Part model, mm, in its own coordinate system. A direction names the side the tool comes from. Round coordinates to 2 decimals unless told otherwise and drop trailing zeros. Order: outer loops, then holes, each group sorted by start corner. A loop starts at its lowest first (then second) coordinate and runs counter-clockwise, first axis right, second up. Notation, with made-up numbers: M 38.25,-31.5 L 88.25,-31.5 A6 cw 88.25,-27.5 Z; hole C 39,-24.75 d10. An arc over 180 degrees is marked long. One line per question, with ' | ' between items.
from build123d import *

# Parameters (mm, degrees)
F0_W     = 150
F0_H     = 125
F0_R     = 20
F1_DEPTH = 5
F2_R     = 10
F4_D     = 8.5
F4_DEPTH = 24.5
F4_TIP   = 2.5536576309
F6_DEPTH = 10.001


with BuildPart() as f1:
    # F0 (on Front) → F1 (new body, symmetric)
    with BuildSketch(Plane.XZ):
        Rectangle(F0_W, F0_H)
        Circle(F0_R, mode=Mode.SUBTRACT)
    extrude(amount=F1_DEPTH, both=True)

    # F2
    f2_edges = [f1.edges().sort_by_distance(p)[0] for p in [
        (-75, 0, 62.5),
        (75, 0, 62.5),
        (75, 0, -62.5),
        (-75, 0, -62.5),
    ]]
    fillet(f2_edges, radius=F2_R)

    # F4
    with Locations(Plane.XZ.offset(5)):
        with Locations((-49.5, 0), (49.5, 0)):
            Hole(F4_D / 2, depth=F4_DEPTH)
            with Locations((0, 0, -(F4_DEPTH + F4_TIP / 2))):  # 118° drill point
                Cone(0, F4_D / 2, F4_TIP, mode=Mode.SUBTRACT)

    # F5 (on face) → F6 (cut, through all)
    with BuildSketch(Plane.XZ.offset(5)):
        with BuildLine():
            ThreePointArc((-37.5, 53), (-43, 47.5), (-37.5, 42))
            Line((-37.5, 42), (37.5, 42))
            ThreePointArc((37.5, 42), (43, 47.5), (37.5, 53))
            Line((37.5, 53), (-37.5, 53))
        make_face()
        with BuildLine():
            ThreePointArc((37.5, -53), (43, -47.5), (37.5, -42))
            Line((37.5, -42), (-37.5, -42))
            ThreePointArc((-37.5, -42), (-43, -47.5), (-37.5, -53))
            Line((-37.5, -53), (37.5, -53))
        make_face()
    extrude(amount=-F6_DEPTH, mode=Mode.SUBTRACT)


solid = f1.part
1) Saw through at A-A (z = 47.5). List the corners of the cut face in (x, y).
The answers:
outline: M -75,-5 L -43,-5 L -43,5 L -75,5 Z; M 43,-5 L 75,-5 L 75,5 L 43,5 Z
2) Which spindle directions (+Z, -Z, +X, -X, +Y, -Y) get a long thin tool onto all of the face, cutting with end or side? Do faces 1 (the face through (-1, 0, -62.5)), 2 (the face through (-1, 0, -53)). Say none if no direction does.
The answers:
face 1: -Z, +X, -X, +Y, -Y | face 2: +Y, -Y
3) Saw through at C-C (x = 33). List the corners of the cut face in (y, z).
The answers:
outline: M -5,-62.5 L 5,-62.5 L 5,-53 L -5,-53 Z; M -5,-42 L 5,-42 L 5,42 L -5,42 Z; M -5,53 L 5,53 L 5,62.5 L -5,62.5 Z
4) Saw through at D-D (y = 1.5). List the corners of the cut face in (x, z), plus the area to 3 significant figures.
The answers:
outline: M -75,-52.5 A10 ccw -65,-62.5 L 65,-62.5 A10 ccw 75,-52.5 L 75,52.5 A10 ccw 65,62.5 L -65,62.5 A10 ccw -75,52.5 Z; hole C -49.5,0 d8.5; hole M -37.5,-53 L 37.5,-53 A5.5 ccw 37.5,-42 L -37.5,-42 A5.5 ccw Z; hole M -37.5,42 L 37.5,42 A5.5 ccw 37.5,53 L -37.5,53 A5.5 ccw Z; hole C 0,0 d40; hole C 49.5,0 d8.5 | area: 15,500 mm²
5) Two-plate mould, pull along Z, no slides. Class faces 3 (the face through (-43, -0.1, -47.4)), 4 (the face through (72.15, -0.07, -59.49)), 5 (the face through (75, 0, -1)), 6 (the face through (43, -0.1, 47.4)): released by +Z, released by -Z, zero draft, split by the parting line, or undercut.
The answers:
face 3: undercut | face 4: released by -Z | face 5: zero draft | face 6: undercut
6) Probe line 1 (Z direction, x = 0, y = 1.25); line 2 (Z direction, x = 49.5, y = -1); line 3 (Z direction, x = -4, y = 0.5). List the from-to ranges inside material, lowest first. Write a range as [from, to].
The answers:
line 1: z = [-62.5, -53], [-42, -20], [20, 42], [53, 62.5] | line 2: z = [-62.5, -4.25], [4.25, 62.5] | line 3: z = [-62.5, -53], [-42, -19.6], [19.6, 42], [53, 62.5]
7) Saw through at B-B (x = -51.5). List the corners of the cut face in (y, z), plus the area to 4 significant figures.
The answers:
outline: M -5,-62.5 L 5,-62.5 L 5,-3.75 L -5,-3.75 Z; M -5,3.75 L 5,3.75 L 5,62.5 L -5,62.5 Z | area: 1,175 mm²
